from build123d import *

# Parameters (mm, degrees)
SKETCH1_R           = 1.0922
BOSS_EXTRUDE1_DEPTH = 3.175


with BuildPart() as part:
    # Sketch1 → Boss-Extrude1 (new body)
    with BuildSketch(Plane.XY):
        Polygon((32.995567884, 19.05), (0, 38.1), (-32.995567884, 19.05), (-32.995567884, -19.05), (0, -38.1), (32.995567884, -19.05), align=None)
        with Locations((-29.696011096, 17.145)):
            Circle(SKETCH1_R, mode=Mode.SUBTRACT)
        with Locations((0, 34.29)):
            Circle(SKETCH1_R, mode=Mode.SUBTRACT)
        with Locations((29.696011096, 17.145)):
            Circle(SKETCH1_R, mode=Mode.SUBTRACT)
        with Locations((29.696011096, -17.145)):
            Circle(SKETCH1_R, mode=Mode.SUBTRACT)
        with Locations((0, -34.29)):
            Circle(SKETCH1_R, mode=Mode.SUBTRACT)
        with Locations((-29.696011096, -17.145)):
            Circle(SKETCH1_R, mode=Mode.SUBTRACT)
        Polygon((26.396454307, 15.24), (0, 30.48), (-26.396454307, 15.24), (-26.396454307, -15.24), (0, -30.48), (26.396454307, -15.24), align=None, mode=Mode.SUBTRACT)
    extrude(amount=BOSS_EXTRUDE1_DEPTH)


solid = part.part
Part model, mm, in its own coordinate system. A direction names the side the tool comes from. Give positions to 0.01 mm unless a question says otherwise; leave off trailing zeros. Loops run counter-clockwise (first coordinate to the right, second up) from the corner with the lowest first, then second, coordinate; pieces in that order, holes last. Notation, with made-up numbers: M -12,3 L 2,3 A14 cw 2,14 Z; hole C -19,-37.5 d1. An arc over 180 degrees is marked long. Put each result on its own line as item: value. Start each with the question number.
1) Flat gauge pin, fed straight in: pin 1 (1 mm diameter, centred on x = -7.5, z = 0.5, fed in from -Y). Where does the tip first touch, or does it go through?
2) Saw through at C-C (z = 1.8). List the corners of the cut face in (x, y) (3 decimals), then the cut area to 3 significant figures.
3) 3-axis set-ups, long thin cutter, end or side, ignore diameter. For faces 1 (the flat face through (13.383, 22.753, 1.565)), 2 (the flat face through (-10, -25, 0)): which of +Z, -Z, +X, -X, +Y, -Y reach the whole face in a straight line?
4) Probe probe 1 along Y at (x, z) = (0, 1.05); probe 2 along X at (y, z) = (-12.5, 1.15); probe 3 along X at (y, z) = (-17.5, 0.85). List the from-to ranges inside material, lowest first.
5) Saw through at A-A (y = 11). List the corners of the cut face in (x, z) (3 decimals).
6) Pull direction Y, two halves, no side cores. Call faces 3 (the cylindrical face through (30.74, 17.47, 1.57)), 4 (the cylindrical face through (-0.142, -33.207, 1.565)), 5 (the flat face through (16.73, 28.44, 1.57)), 6 (the flat face through (-10, -25, 3.175)): +Y half, -Y half, draft (parallel to the pull), parting line (faces both ways), or undercut.
7) Saw through at B-B (x = 15). List the corners of the cut face in (y, z) (3 decimals), then the cut area to 3 significant figures.
Numbers:
1. pin 1: y = -34.06
2. outline: M -32.996,-19.05 L 0,-38.1 L 32.996,-19.05 L 32.996,19.05 L 0,38.1 L -32.996,19.05 Z; hole C -29.696,-17.145 d2.184; hole C -29.696,17.145 d2.184; hole M -26.396,-15.24 L 0,-30.48 L 26.396,-15.24 L 26.396,15.24 L 0,30.48 L -26.396,15.24 Z; hole C 0,-34.29 d2.184; hole C 0,34.29 d2.184; hole C 29.696,-17.145 d2.184; hole C 29.696,17.145 d2.184
2. area: 1,340 mm^2
3. face 1: +Z, -Z
3. face 2: -Z, +X, -X, +Y, -Y
4. probe 1: -38.1 to -35.38, -33.2 to -30.48, 30.48 to 33.2, 35.38 to 38.1
4. probe 2: -33 to -26.4, 26.4 to 33
4. probe 3: -33 to -30.73, -28.66 to -22.48, 22.48 to 28.66, 30.73 to 33
5. outline: M -32.996,0 L -26.396,0 L -26.396,3.175 L -32.996,3.175 Z; M 26.396,0 L 32.996,0 L 32.996,3.175 L 26.396,3.175 Z
6. face 3: undercut
6. face 4: undercut
6. face 5: +Y half
6. face 6: draft
7. outline: M -29.44,0 L -21.82,0 L -21.82,3.175 L -29.44,3.175 Z; M 21.82,0 L 29.44,0 L 29.44,3.175 L 21.82,3.175 Z
7. area: 48.4 mm^2
